Verification items for this drawing (mm, ordinates from the low corner). Coordinates: 2 decimals unless noted, no trailing zeros. Write each loop counter-clockwise with the first axis right and the second up, starting at its lowest first coordinate (ties: lowest second). Pieces come first, ordered by that corner, then holes. Notation, with made-up numbers: (9, 52.5) -> (57, 52.5) arc R18 cw to (57, 69.5) -> close; hole circle Ø1 at (65.5, -7). An arc over 180 degrees is marked (long way). One line per question, with ' | ' between items.
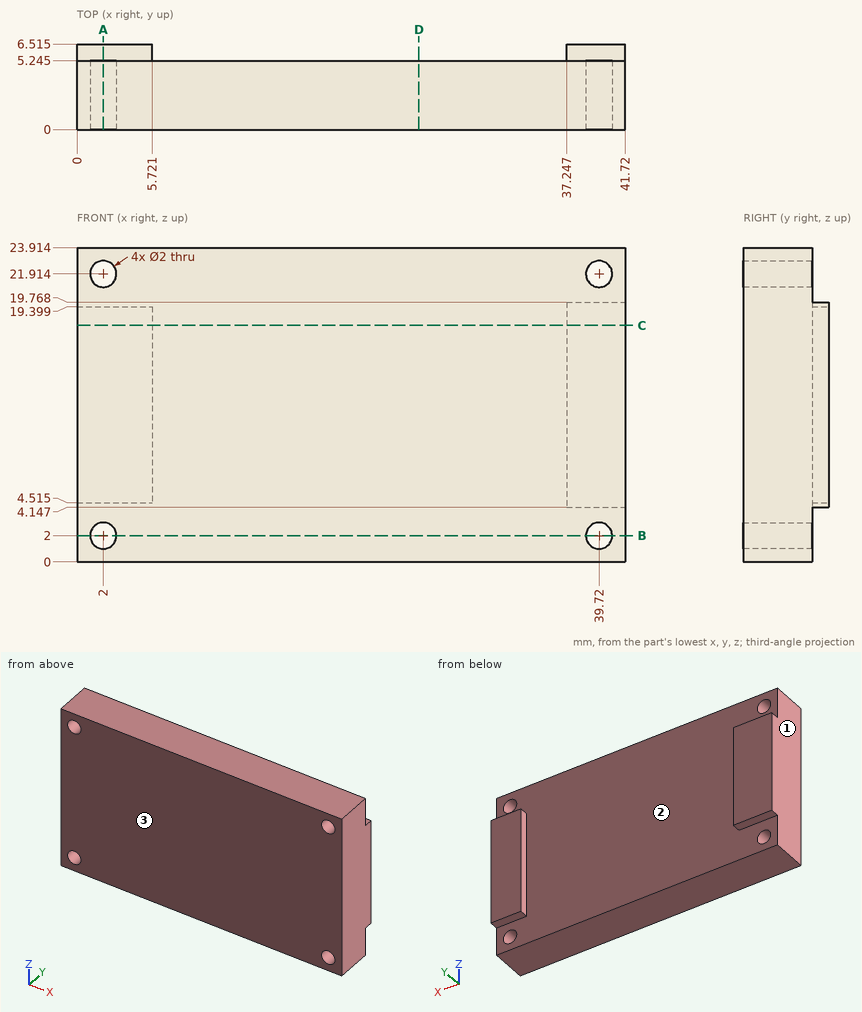
(1) Cross-section at D-D (x = 26). Record the cut outline in (y, z) (1 decimal).
Answers below:
outline: (0, 0) -> (5.2, 0) -> (5.2, 23.9) -> (0, 23.9) -> close
(2) Cross-section at B-B (z = 2). Record the cut outline in (x, y) (1 decimal), plus the area to 3 significant figures.
Answers below:
outline: (0, 0) -> (1, 0) -> (1, 5.2) -> (0, 5.2) -> close; (3, 0) -> (38.7, 0) -> (38.7, 5.2) -> (3, 5.2) -> close; (40.7, 0) -> (41.7, 0) -> (41.7, 5.2) -> (40.7, 5.2) -> close | area: 198 mm²
(3) Depth check by flat-ended pin: P1, Ø1, axis at x = 4, y = 6, coming from the +Z side; P2, Ø0.6, axis at x = 39, y = 6, coming from the -Z side; P3, Ø1, axis at x = 2.5, y = 6, coming from the -Z side (1 decimal); P4, Ø1.8, axis at x = 2, z = 2, coming from the +Y side. Enter the tip coordinate at first touch or a pass-through.
Answers below:
P1: stops at z = 19.4 | P2: stops at z = 4.15 | P3: stops at z = 4.5 | P4: passes through
(4) Draft check along X on the marked faces 1, 2 and 3. Enter one of: pulls with the +X half, pulls with the -X half, needs draft (parallel to the pull), parting line crosses it, or undercut.
Answers below:
face 1: pulls with the -X half | face 2: undercut | face 3: needs draft
(5) Cross-section at C-C (z = 18). Record the cut outline in (x, y) (1 decimal).
Answers below:
outline: (0, 0) -> (41.7, 0) -> (41.7, 6.5) -> (37.2, 6.5) -> (37.2, 5.2) -> (5.7, 5.2) -> (5.7, 6.5) -> (0, 6.5) -> close
(6) Cross-section at A-A (x = 2). Record the cut outline in (y, z) (1 decimal), plus the area to 3 significant figures.
Answers below:
outline: (0, 0) -> (5.2, 0) -> (5.2, 1) -> (0, 1) -> close; (0, 3) -> (5.2, 3) -> (5.2, 4.5) -> (6.5, 4.5) -> (6.5, 19.4) -> (5.2, 19.4) -> (5.2, 20.9) -> (0, 20.9) -> close; (0, 22.9) -> (5.2, 22.9) -> (5.2, 23.9) -> (0, 23.9) -> close | area: 123 mm²
(7) Material ranges on line 1 (X direction, y = 2.95, z = 2); line 2 (X direction, y = 1.25, z = 2.25); line 3 (Y direction, x = 21.5, z = 7) (1 decimal), recorded low to high.
Answers below:
line 1: x = 0 to 1, 3 to 38.72, 40.72 to 41.72 | line 2: x = 0 to 1.03, 2.97 to 38.75, 40.69 to 41.72 | line 3: y = 0 to 5.2
